CAD build for the part. Positions are in the model's coordinates, mm. Give positions to 0.01 mm unless a question says otherwise; leave off trailing zeros. Loops run counter-clockwise (first coordinate to the right, second up) from the corner with the lowest first, then second, coordinate; pieces in that order, holes last. Notation, with made-up numbers: (63, -21) -> (85, -21) arc R18 cw to (85, 6) -> close; hole circle Ø7 at (56.25, -28.5). An arc over 180 degrees is marked (long way). Write each question's results on one line, items separated by ' | '. Start each with the question number.
```python
from build123d import *

# Parameters (mm, degrees)
F0_R     = 6.35
F1_DEPTH = 101.5999987721
F2_R     = 12.7
F3_DEPTH = 12.7


# Not quite as in the source:
# - a fillet or chamfer that OpenCascade refuses, or shapes differently, is made with other operations: its cross-section is extruded or revolved along the edge and cut away or added


with BuildPart() as f1:
    # F0 (on Front) → F1 (new body)
    with BuildSketch(Plane.XZ):
        Circle(F0_R)
    extrude(amount=-F1_DEPTH)

    # F2 (on face) + F0 (on Front) → F3 (join)
    with BuildSketch(Plane.XZ):
        Circle(F2_R)
    with BuildSketch(Plane.XZ):
        Circle(F0_R)
    extrude(amount=F3_DEPTH)

    # F4: fillet of radius 12.7 on 1 edges, made by hand

    # F4_s1 → F4_t2 (revolve, cut)
    with BuildSketch(Plane.XY):
        with BuildLine():
            add(Edge.make_bspline(
                [(12.7, 0), (12.7, -12.7), (0, -12.7)],
                knots=[0, 0, 0, 1, 1, 1], degree=2, weights=[1, 1, 1]))
            Line((0, -12.7), (12.7, -12.7))
            Line((12.7, -12.7), (12.7, 0))
        make_face()
    revolve(axis=Axis((0, -12.7, 0), (0, -1, 0)), mode=Mode.SUBTRACT)


solid = f1.part
```
Q1. Drop flat-ended pins along their axis: pin 1 (5 mm diameter, centred on x = 3.5, y = 74, fed in from +Z); pin 2 (3 mm diameter, centred on x = 0, z = 10, fed in from -Y); pin 3 (10 mm diameter, centred on x = 2.5, z = 6.5, fed in from -Y). Give the stop position or say it passes through.
Q2. Wall check: L1, parallel to X at y = 74, z = 0.25; L2, parallel to Y at x = -0.5, z = -3.25; L3, parallel to X at y = 20.5, z = -4.25. Give the ranges that are in metal, low to high.
Q3. Saw through at A-A, the plane y = 27. List the corners of the cut face in (x, z), then the cut area to 3 significant figures.
Q4. Mould opens along Z. For faces 1 (the face through (3, 0, 6)), 2 (the face through (-1.38, 50.09, -6.2)) say: pulls with the +Z half, pulls with the -Z half, needs draft (parallel to the pull), parting line crosses it, or undercut.
Answer block:
1) pin 1: stops at z = 6.27 | pin 2: stops at y = -10.41 | pin 3: stops at y = -12.62
2) L1: x = -6.35 to 6.35 | L2: y = -12.45 to 101.6 | L3: x = -4.72 to 4.72
3) outline: circle Ø12.7 at (0, 0) | area: 127 mm2
4) face 1: needs draft | face 2: parting line crosses it
